Could you check a few things on this model? Use its own coordinates, in mm. Face numbers are marked on the shaded views. A direction names the side the tool comes from. Round coordinates to 2 decimals unless told otherwise and drop trailing zeros. Loops run counter-clockwise (first coordinate to the right, second up) from the corner with the lowest first, then second, coordinate; pieces in that order, holes last. Notation, with made-up numbers: (-37, 60.5) -> (-30, 60.5) arc R27 ccw to (-30, 96.5) -> close; hole circle Ø3 at (-27.75, -31.5). An arc over 180 degrees is marked (long way). One line per item, written item: value.
```python
from build123d import *

# Parameters (mm, degrees)
SKETCH1_R           = 25.4
BOSS_EXTRUDE1_DEPTH = 6
SKETCH4_R           = 9.5
BOSS_EXTRUDE2_DEPTH = 6
CUT_EXTRUDE1_REACH  = 39.872
SKETCH6_R           = 3


with BuildPart() as part:
    # Sketch1 → Boss-Extrude1 (new body)
    with BuildSketch(Plane.XY):
        Circle(SKETCH1_R)
    extrude(amount=BOSS_EXTRUDE1_DEPTH)

    # Sketch4 → Boss-Extrude2 (add)
    with BuildSketch(Plane.XY.offset(6)):
        Circle(SKETCH4_R)
    extrude(amount=BOSS_EXTRUDE2_DEPTH)

    # Sketch6 → Cut-Extrude1 (cut, up to next)
    with BuildSketch(Plane.XY, mode=Mode.PRIVATE) as cut_extrude1_sk1:
        Circle(SKETCH6_R)
    cut_extrude1_tool1 = extrude(cut_extrude1_sk1.sketch, amount=CUT_EXTRUDE1_REACH, mode=Mode.PRIVATE) & part.part
    add(cut_extrude1_tool1.solids().sort_by_distance((0, 0, 0))[0], mode=Mode.SUBTRACT)


solid = part.part
```
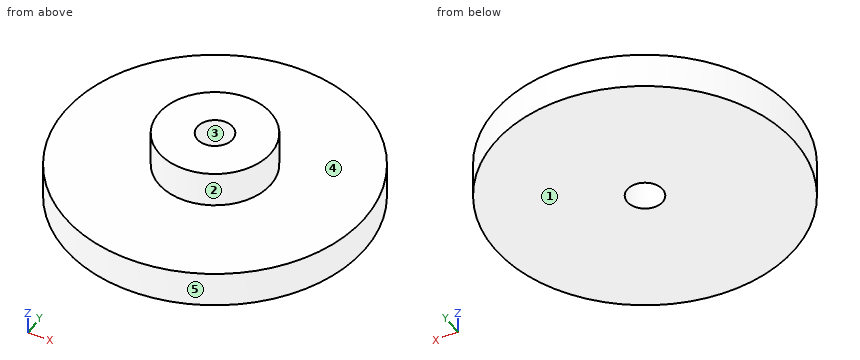
(1) Imagine slicing it at C-C on z = 3.75. Write out the boundary of the cut face in (x, y).
Results below:
outline: circle Ø50.8 at (0, 0); hole circle Ø6 at (0, 0)
(2) On a 3-axis mill with a long thin cutter (end or side, diameter ignored), from which of +Z, -Z, +X, -X, +Y, -Y can I reach the whole of each face in a straight line? I mean the marked faces 1 and 2. Say none if no direction works.
Results below:
face 1: -Z, +X, -X, +Y, -Y
face 2: +Z
(3) Imagine slicing it at A-A on x = 0. Write out the boundary of the cut face in (y, z).
Results below:
outline: (-25.4, 0) -> (-3, 0) -> (-3, 12) -> (-9.5, 12) -> (-9.5, 6) -> (-25.4, 6) -> close; (3, 0) -> (25.4, 0) -> (25.4, 6) -> (9.5, 6) -> (9.5, 12) -> (3, 12) -> close
(4) We'd pull the mould along Y, two halves only. Please class the marked faces 3, 4 and 5: +Y half, -Y half, draft (parallel to the pull), parting line (faces both ways), or undercut.
Results below:
face 3: undercut
face 4: draft
face 5: parting line
(5) For pin 1 Ø1.5 at (x, z) = (0.5, 2.5) entering from -Y; pin 2 Ø2 at (x, z) = (6, 3.5) entering from +Y; pin 3 Ø1.5 at (x, y) = (9.5, -20) entering from +Z, each with a flat end and sliding along its axis, tell me the tip position at first contact or that it passes through.
Results below:
pin 1: stops at y = -25.4
pin 2: stops at y = 24.9
pin 3: stops at z = 6
(6) Please list where these lines run through material, in increasing order: L1, parallel to Y at x = 0, z = 2.5; L2, parallel to Y at x = 0, z = 6.5; L3, parallel to Z at x = 9.5, y = -8.
Results below:
L1: y = -25.4 to -3, 3 to 25.4
L2: y = -9.5 to -3, 3 to 9.5
L3: z = 0 to 6
(7) Imagine slicing it at D-D on x = 6. Write out the boundary of the cut face in (y, z).
Results below:
outline: (-24.68, 0) -> (24.68, 0) -> (24.68, 6) -> (7.37, 6) -> (7.37, 12) -> (-7.37, 12) -> (-7.37, 6) -> (-24.68, 6) -> close
